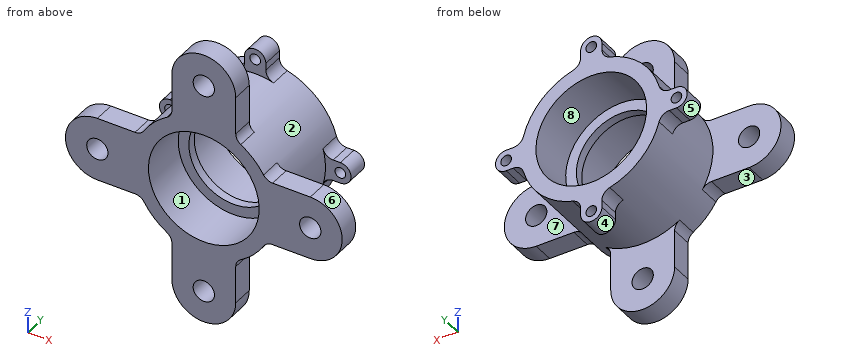
from build123d import *

# Parameters (mm, degrees)
SKETCH2_R           = 2.5
BOSS_EXTRUDE1_DEPTH = 10
SKETCH3_R           = 5
BOSS_EXTRUDE2_DEPTH = 10
FILLET1_R           = 5


with BuildPart() as part:
    # Sketch1 → Revolve1 (revolve)
    with BuildSketch(Plane.XY, mode=Mode.PRIVATE) as revolve1_sk:
        Polygon((26, 24), (26, 2), (21, 2), (21, -2), (26, -2), (26, -24), (33, -24), (33, 24), align=None)
    revolve(revolve1_sk.sketch.rotate(Axis((0, 27.182366668, 0), (0, -1, 0)), 90), axis=Axis((0, 27.182366668, 0), (0, -1, 0)))  # turned: the seam where the file's is

    # Sketch2 → Boss-Extrude1 (add)
    with BuildSketch(Plane.XZ.offset(-24)):
        with BuildLine():
            Line((5, 40), (5, 32.619012861))
            ThreePointArc((5, 32.619012861), (0, 33), (-5, 32.619012861))
            Line((-5, 32.619012861), (-5, 40))
            ThreePointArc((-5, 40), (0, 45), (5, 40))
        make_face()
        with Locations(Location((0, 40, 0), (0, 0, 270))):  # turned: the seam where the file's is
            Circle(SKETCH2_R, mode=Mode.SUBTRACT)
        with BuildLine():
            Line((40, -5), (32.619012861, -5))
            ThreePointArc((32.619012861, -5), (33, 0), (32.619012861, 5))
            Line((32.619012861, 5), (40, 5))
            ThreePointArc((40, 5), (45, 0), (40, -5))
        make_face()
        with Locations(Location((40, 0, 0), (0, 0, 270))):  # turned: the seam where the file's is
            Circle(SKETCH2_R, mode=Mode.SUBTRACT)
        with BuildLine():
            Line((-5, -40), (-5, -32.619012861))
            ThreePointArc((-5, -32.619012861), (0, -33), (5, -32.619012861))
            Line((5, -32.619012861), (5, -40))
            ThreePointArc((5, -40), (0, -45), (-5, -40))
        make_face()
        with Locations(Location((0, -40, 0), (0, 0, 270))):  # turned: the seam where the file's is
            Circle(SKETCH2_R, mode=Mode.SUBTRACT)
        with BuildLine():
            Line((-40, 5), (-32.619012861, 5))
            ThreePointArc((-32.619012861, 5), (-33, 0), (-32.619012861, -5))
            Line((-32.619012861, -5), (-40, -5))
            ThreePointArc((-40, -5), (-45, 0), (-40, 5))
        make_face()
        with Locations(Location((-40, 0, 0), (0, 0, 270))):  # turned: the seam where the file's is
            Circle(SKETCH2_R, mode=Mode.SUBTRACT)
    extrude(amount=BOSS_EXTRUDE1_DEPTH)

    # Sketch3 → Boss-Extrude2 (add)
    with BuildSketch(Plane(origin=(0, -24, 0), x_dir=(-1, 0, 0), z_dir=(0, 1, 0))):
        with BuildLine():
            Line((-15, 50), (-15, 29.393876913))
            ThreePointArc((-15, 29.393876913), (0, 33), (15, 29.393876913))
            Line((15, 29.393876913), (15, 50))
            ThreePointArc((15, 50), (0, 65), (-15, 50))
        make_face()
        with Locations(Location((0, 50, 0), (0, 0, 90))):  # turned: the seam where the file's is
            Circle(SKETCH3_R, mode=Mode.SUBTRACT)
        with BuildLine():
            Line((50, 15), (29.393876913, 15))
            ThreePointArc((29.393876913, 15), (33, 0), (29.393876913, -15))
            Line((29.393876913, -15), (50, -15))
            ThreePointArc((50, -15), (65, 0), (50, 15))
        make_face()
        with Locations(Location((50, 0, 0), (0, 0, 90))):  # turned: the seam where the file's is
            Circle(SKETCH3_R, mode=Mode.SUBTRACT)
        with BuildLine():
            Line((15, -50), (15, -29.393876913))
            ThreePointArc((15, -29.393876913), (0, -33), (-15, -29.393876913))
            Line((-15, -29.393876913), (-15, -50))
            ThreePointArc((-15, -50), (0, -65), (15, -50))
        make_face()
        with Locations(Location((0, -50, 0), (0, 0, 90))):  # turned: the seam where the file's is
            Circle(SKETCH3_R, mode=Mode.SUBTRACT)
        with BuildLine():
            Line((-50, -15), (-29.393876913, -15))
            ThreePointArc((-29.393876913, -15), (-33, 0), (-29.393876913, 15))
            Line((-29.393876913, 15), (-50, 15))
            ThreePointArc((-50, 15), (-65, 0), (-50, -15))
        make_face()
        with Locations(Location((-50, 0, 0), (0, 0, 90))):  # turned: the seam where the file's is
            Circle(SKETCH3_R, mode=Mode.SUBTRACT)
    extrude(amount=BOSS_EXTRUDE2_DEPTH)

    # Fillet1
    fillet1_edges = [part.edges().sort_by_distance(p)[0] for p in [
        (-15, -19, -29.393876913),
        (15, -19, -29.393876913),
        (29.393876913, -19, -15),
        (29.393876913, -19, 15),
        (-5, 19, 32.619012861),
        (5, 19, 32.619012861),
        (32.619012861, 19, 5),
        (32.619012861, 19, -5),
        (5, 19, -32.619012861),
        (-5, 19, -32.619012861),
        (-32.619012861, 19, -5),
        (-32.619012861, 19, 5),
        (15, -19, 29.393876913),
        (-15, -19, 29.393876913),
        (-29.393876913, -19, 15),
        (-29.393876913, -19, -15),
    ]]
    fillet(fillet1_edges, radius=FILLET1_R)


solid = part.part
Can you work these out from the model? Positions are in its coordinate system, mm. Face numbers are marked on the shaded views. A direction names the side the tool comes from. Round coordinates to 2 decimals unless told otherwise and drop trailing zeros. Write each loop counter-clockwise with the first axis right and the second up, starting at its lowest first coordinate (ties: lowest second). Pieces come first, ordered by that corner, then holes. Notation, with made-up numbers: M 23,19.5 L 71,19.5 A17 cw 71,44.5 Z; hole C 36,82 d8. An arc over 180 degrees is marked long. Use a Markdown table: item, result.
Item 1: Which directions (+Z, -Z, +X, -X, +Y, -Y) give clear straight access to the entire face, cutting with the end or side of a thin tool? Please do the marked faces 1, 2, 3, 4 and 5.
Found:
| item | result |
|---|---|
| face 1 | -Y |
| face 2 | none |
| face 3 | -Z, -X, +Y, -Y |
| face 4 | -Z, +Y |
| face 5 | -X, +Y |
Item 2: I want a section at D-D (y = 8.5). List the corners of the cut face in (x, z) for me.
Found:
| item | result |
|---|---|
| outline | C 0,0 d66; hole C 0,0 d52 |
Item 3: I want a section at A-A (y = 20.5). State how many separate pieces and enclosed holes the cut face has, and give its area (3 significant figures).
Found:
| item | result |
|---|---|
| separate pieces | 1 |
| enclosed holes | 5 |
| area | 1,690 mm2 |
Item 4: If I drill on line 1 along X through (y, z) = (-20, 0); line 2 along X through (y, z) = (16, 0); line 3 along X through (y, z) = (18.25, -40), over which ranges is the centre line in solid material (lowest first)? Write a range as [from, to].
Found:
| item | result |
|---|---|
| line 1 | x = [-65, -55], [-45, -26], [26, 45], [55, 65] |
| line 2 | x = [-45, -42.5], [-37.5, -26], [26, 37.5], [42.5, 45] |
| line 3 | x = [-5, -2.5], [2.5, 5] |
Item 5: I want a section at B-B (x = -52). List the corners of the cut face in (y, z) for me, and give its area (3 significant figures).
Found:
| item | result |
|---|---|
| outline | M -24,-14.87 L -14,-14.87 L -14,-4.58 L -24,-4.58 Z; M -24,4.58 L -14,4.58 L -14,14.87 L -24,14.87 Z |
| area | 206 mm2 |
Item 6: For pin 1 Ø1 at (y, z) = (21, -38.5) entering from +X; pin 2 Ø3 at (x, y) = (40.5, -19.5) entering from +Z; pin 3 Ø9 at (x, z) = (0, -50) entering from +Y; pin 4 Ø10.5 at (x, z) = (-6, -51) entering from +Y, each with a flat end and sliding along its axis, tell me the tip position at first contact or that it passes through.
Found:
| item | result |
|---|---|
| pin 1 | stops at x = 5 |
| pin 2 | stops at z = 15 |
| pin 3 | passes through |
| pin 4 | stops at y = -14 |
Item 7: We'd pull the mould along Z, two halves only. Please class the marked faces 6, 7 and 8: released by +Z, released by -Z, zero draft, split by the parting line, or undercut.
Found:
| item | result |
|---|---|
| face 6 | split by the parting line |
| face 7 | zero draft |
| face 8 | undercut |
